The model under review builds one solid part; all positions refer to its coordinate system, in mm. Coordinates: 2 decimals unless noted, no trailing zeros. Order: outer loops, then holes, each group sorted by start corner. A loop starts at its lowest first (then second) coordinate and runs counter-clockwise, first axis right, second up. Notation, with made-up numbers: (-21.5, 15.5) - (36.5, 15.5) arc R8 ccw to (36.5, 27.5) - close; hole circle Ø1 at (11.25, -20.5). An arc over 180 degrees is marked (long way). Answer in a Markdown table with one row per item.
```python
from build123d import *

# Parameters (mm, degrees)
SKETCH1_R           = 2.5527
SKETCH1_R_2         = 14.2875
SKETCH1_R_3         = 2.286
BOSS_EXTRUDE1_DEPTH = 1.5875
SKETCH2_W           = 61.9125
SKETCH2_H           = 218.44
CUT_EXTRUDE1_DEPTH  = 2.5875
CHAMFER1_SIZE       = 88.9


with BuildPart() as part:
    # Sketch1 → Boss-Extrude1 (new body)
    with BuildSketch(Plane.XY):
        with BuildLine():
            Line((-182.5625, -359.614215072), (74.6125, -359.614215072))
            Line((74.6125, -359.614215072), (74.6125, 100.125784928))
            Line((74.6125, 100.125784928), (-184.15, 100.125784928))
            Line((-184.15, 100.125784928), (-184.15, -323.589680411))
            ThreePointArc((-184.15, -323.589680411), (-183.358351266, -324.237998925), (-182.5625, -324.881151609))
            Line((-182.5625, -324.881151609), (-182.5625, -359.614215072))
        make_face()
        with Locations((-84.1375, -227.673915072)):
            Circle(SKETCH1_R, mode=Mode.SUBTRACT)
        with Locations((-109.5375, -202.273915072)):
            Circle(SKETCH1_R, mode=Mode.SUBTRACT)
        with Locations((-84.1375, -202.273915072)):
            Circle(SKETCH1_R_2, mode=Mode.SUBTRACT)
        with Locations((-84.1375, -176.873915072)):
            Circle(SKETCH1_R, mode=Mode.SUBTRACT)
        with Locations((-58.7375, -202.273915072)):
            Circle(SKETCH1_R, mode=Mode.SUBTRACT)
        with Locations((-26.369714503, -340.552266808)):
            Circle(SKETCH1_R_3, mode=Mode.SUBTRACT)
        with Locations((7.450966894, -320.88914315)):
            Circle(SKETCH1_R_3, mode=Mode.SUBTRACT)
        with Locations((35.030045629, -293.14258772)):
            Circle(SKETCH1_R_3, mode=Mode.SUBTRACT)
        with Locations((54.488053063, -259.203482417)):
            Circle(SKETCH1_R_3, mode=Mode.SUBTRACT)
        with Locations((64.498958145, -221.384721179)):
            Circle(SKETCH1_R_3, mode=Mode.SUBTRACT)
        with BuildLine():
            Line((73.025, -206.741987336), (73.025, -202.273915072))
            Line((73.025, -202.273915072), (73.025, -197.805842809))
            ThreePointArc((73.025, -197.805842809), (73.0885, -202.273915072), (73.025, -206.741987336))
        make_face(mode=Mode.SUBTRACT)
        with Locations((62.145886508, -182.799411028)):
            Circle(SKETCH1_R_3, mode=Mode.SUBTRACT)
        with Locations((-158.413638358, -69.463111493)):
            Circle(SKETCH1_R_3, mode=Mode.SUBTRACT)
        with Locations((-135.03744834, -108.096679976)):
            Circle(SKETCH1_R_3, mode=Mode.SUBTRACT)
        with Locations((-102.458679377, -139.363638358)):
            Circle(SKETCH1_R_3, mode=Mode.SUBTRACT)
        with Locations((-170.994200713, -26.095746755)):
            Circle(SKETCH1_R_3, mode=Mode.SUBTRACT)
        with Locations((5.529920705, -85.065386628)):
            Circle(SKETCH1_R_3, mode=Mode.SUBTRACT)
        with Locations((32.810376845, -112.26680659)):
            Circle(SKETCH1_R_3, mode=Mode.SUBTRACT)
        with Locations((52.121028445, -145.602062252)):
            Circle(SKETCH1_R_3, mode=Mode.SUBTRACT)
        with Locations((0, -25.4)):
            Circle(SKETCH1_R, mode=Mode.SUBTRACT)
        with Locations((-25.4, 0)):
            Circle(SKETCH1_R, mode=Mode.SUBTRACT)
        Circle(SKETCH1_R_2, mode=Mode.SUBTRACT)
        with Locations((0, 25.4)):
            Circle(SKETCH1_R, mode=Mode.SUBTRACT)
        with Locations((25.4, 0)):
            Circle(SKETCH1_R, mode=Mode.SUBTRACT)
    extrude(amount=BOSS_EXTRUDE1_DEPTH)

    # Sketch2 → Cut-Extrude1 (cut, through all)
    with BuildSketch(Plane.XY.offset(1.5875)):
        with Locations((-153.19375, -250.394215072)):
            Rectangle(SKETCH2_W, SKETCH2_H)
    extrude(amount=-CUT_EXTRUDE1_DEPTH, mode=Mode.SUBTRACT)

    # Chamfer1
    chamfer1_edges = [part.edges().sort_by_distance(p)[0] for p in [
        (74.6125, -359.614215072, 0.79375),
    ]]
    chamfer(chamfer1_edges, length=CHAMFER1_SIZE)


solid = part.part
```
Item 1: Mouldability with a two-part tool opening along X and no side actions: class faces 1 (the face through (-14.274, 0.628, 0.783)), 2 (the face through (-57, -127, 1.588)), 3 (the face through (30.785, -314.542, 0.783)) as +X half, -X half, draft (parallel to the pull), parting line (faces both ways), or undercut.
Check values:
| item | result |
|---|---|
| face 1 | undercut |
| face 2 | draft |
| face 3 | +X half |
Item 2: To check wall thickness, follow line 1 (Y direction, x = -84, z = 1.1); line 2 (Y direction, x = 7.5, z = 0.3); line 3 (Y direction, x = -165.5, z = 1.45). State the ranges of each line that lie inside material, in increasing order. Write a range as from..to.
Check values:
| item | result |
|---|---|
| line 1 | -359.61..-230.22, -225.12..-216.56, -187.99..-179.42, -174.32..100.13 |
| line 2 | -337.83..-323.17, -318.6..-86.22, -83.91..-12.16, 12.16..100.13 |
| line 3 | -141.17..100.13 |
Item 3: We need section A-A, the plane x = -150.5. Write out the cut boundary in (y, z), then the cut area to 3 significant figures.
Check values:
| item | result |
|---|---|
| outline | (-141.17, 0) - (100.13, 0) - (100.13, 1.59) - (-141.17, 1.59) - close |
| area | 383 mm^2 |
